Source: CAD feature listing. Evaluate the final solid. Frame: model axes, mm. Face numbers are marked on the shaded views. A direction names the side the tool comes from. Coordinates: 2 decimals unless noted, no trailing zeros. Loops run counter-clockwise (first coordinate to the right, second up) from the corner with the lowest first, then second, coordinate; pieces in that order, holes last. Notation, with made-up numbers: (80, 12) -> (103, 12) arc R18 cw to (103, 26) -> close; hole circle Ø2 at (54.5, 63.5). An arc over 180 degrees is marked (long way). Answer as CSV lines item,"result".
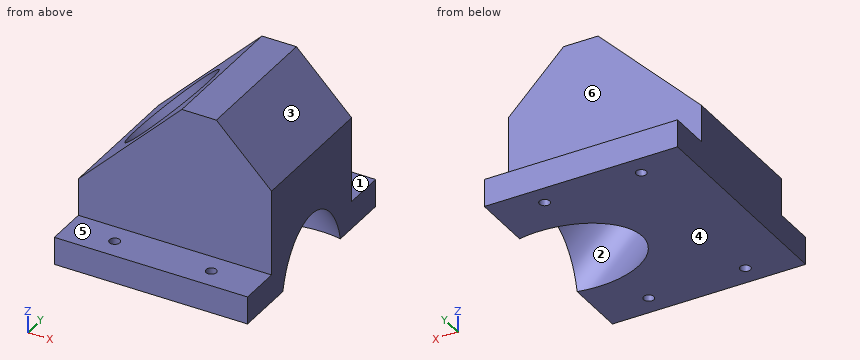
from build123d import *

# Parameters (mm, degrees)
F0_W     = 280
F0_H     = 40
F1_DEPTH = 160
F2_DEPTH = 100
F4_R     = 7.5
F5_R     = 7.5
F6_DEPTH = 40.001
F3_R     = 75
F7_DEPTH = 264.4589361638


with BuildPart() as f1:
    # F0 (on Front) → F1 (new body, symmetric)
    with BuildSketch(Plane.XZ):
        with Locations((0, -102)):
            Rectangle(F0_W, F0_H)
    extrude(amount=F1_DEPTH, both=True)

    # F0 (on Front) → F2 (join, symmetric)
    with BuildSketch(Plane.XZ):
        Polygon((60, 122), (10, 122), (-140, -28), (-140, -82), (140, -82), (140, 42), align=None)
    extrude(amount=F2_DEPTH, both=True)

    # F4 (on face) + F5 (on face) → F6 (cut, through all)
    with BuildSketch(Plane.XY.offset(-82)):
        with Locations((70, 130)):
            Circle(F4_R)
        with Locations((-70, 130)):
            Circle(F4_R)
    with BuildSketch(Plane.XY.offset(-82)):
        with Locations((-70, -130)):
            Circle(F5_R)
        with Locations((70, -130)):
            Circle(F5_R)
    extrude(amount=-F6_DEPTH, mode=Mode.SUBTRACT)

    # F3 (on face) → F7 (cut, through all)
    with BuildSketch(Plane(origin=(-56, 0, 56), x_dir=(0, -1, 0), z_dir=(-0.7071067812, 0, 0.7071067812))):
        with Locations((0, -8.6445035856)):
            Circle(F3_R)
    extrude(amount=-F7_DEPTH, mode=Mode.SUBTRACT)


solid = f1.part
(1) Access query for the marked faces 4, 5 and 6. Directions: +Z, -Z, +X, -X, +Y, -Y. A direction counts if a zero-diameter tool reaches every point of the face in a straight line with its end or side. Return the directions, or none.
Computed values:
face 4,"-Z, +X, -X, +Y, -Y"
face 5,"+Z, +X, -X, -Y"
face 6,"+Z, +X, -X, +Y"
(2) Cut plane D-D (y = 91). Return the cut outline in (x, z).
Computed values:
outline,"(-140, -122) -> (140, -122) -> (140, 42) -> (60, 122) -> (10, 122) -> (-140, -28) -> close"
(3) Cut plane B-B (y = -9). Return the cut outline in (x, z), then the cut area to 3 significant figures.
Computed values:
outline,"(-140, -122) -> (4.48, -122) -> (-114.76, -2.76) -> (-140, -28) -> close; (-9.46, 102.54) -> (140, -46.93) -> (140, 42) -> (60, 122) -> (10, 122) -> close"
area,"20,500 mm^2"
(4) Draft query along X for the marked faces 1, 2 and 3. Return one class per face: released by +X, released by -X, zero draft, split by the parting line, or undercut.
Computed values:
face 1,"zero draft"
face 2,"undercut"
face 3,"released by +X"
(5) Pin query (flat end, axial travel): pin 1 Ø2 at (x, z) = (86, -73) entering from +Y; pin 2 Ø24 at (x, y) = (70, -130) entering from +Z; pin 3 Ø13.5 at (x, y) = (-70, -130) entering from +Z. Return the tip coordinate at first contact, or that it passes through.
Computed values:
pin 1,"y = 100"
pin 2,"z = -82"
pin 3,"through"
(6) Material intervals for L1, parallel to Y at x = 70, z = -104; L2, parallel to Y at x = 70, z = -95; L3, parallel to Z at x = 0, y = -120, sorted ascending. Write a range as [from, to].
Computed values:
L1,"[-160, -137.5], [-122.5, -73.4], [73.4, 122.5], [137.5, 160]"
L2,"[-160, -137.5], [-122.5, -74.45], [74.45, 122.5], [137.5, 160]"
L3,"[-122, -82]"
(7) Cut plane C-C (x = 70). State how many separate pieces and enclosed holes the cut face has, then the cut area to 3 significant figures.
Computed values:
separate pieces,"3"
enclosed holes,"0"
area,"32,100 mm^2"
(8) Cut plane A-A (y = -130). Return the cut outline in (x, z), then the cut area to 3 significant figures.
Computed values:
outline,"(-140, -122) -> (-77.5, -122) -> (-77.5, -82) -> (-140, -82) -> close; (-62.5, -122) -> (62.5, -122) -> (62.5, -82) -> (-62.5, -82) -> close; (77.5, -122) -> (140, -122) -> (140, -82) -> (77.5, -82) -> close"
area,"10,000 mm^2"
